The listing builds one solid part. Answer for the finished solid, in the listing's coordinates (mm). Face numbers are marked on the shaded views. A direction names the side the tool comes from. Give positions to 0.01 mm unless a question says otherwise; leave off trailing zeros. Order: outer loops, then holes, each group sorted by start corner. A loop starts at its lowest first (then second) coordinate and runs counter-clockwise, first axis right, second up. Notation, with made-up numbers: (49.25, -40) - (77.25, -40) arc R22 cw to (77.25, -7) - close; hole circle Ø7 at (61, 35.5). An arc over 180 degrees is marked (long way). Write each question's results on one line, items separated by ' | '. Start each with the question number.
1. Flat-ended cylindrical pins translate along their axes: pin 1 (5 mm diameter, centred on x = -16, y = -20, fed in from +Z); pin 2 (4 mm diameter, centred on x = -14.5, z = 6, fed in from +Y); pin 3 (9 mm diameter, centred on x = -18, y = 18.5, fed in from +Z). Find the tip coordinate at first contact, or state that the pin passes through.
2. Section D-D (z = 8) is taken. Give the vertices of the cut face in (x, y), and give its area (3 significant figures).
3. Section B-B (x = 0) is taken. Give the vertices of the cut face in (y, z) (3 decimals).
4. Which of the six approach directions +Z, -Z, +X, -X, +Y, -Y give full straight-line access (tool end or side, diameter ignored) to the marked faces 1, 2, 3 and 4?
5. Find the intervals of material crossed by L1, parallel to Z at x = 9.5, y = 21; L2, parallel to Z at x = -10, y = 1 (3 decimals); L3, parallel to Z at x = 23, y = -5, in increasing order.
6. Determine the mould class of the marked faces 5, 6, 7 and 8 for opening direction Z: released by +Z, released by -Z, zero draft, split by the parting line, or undercut.
7. Section A-A (z = 0) is taken. Give the vertices of the cut face in (x, y) (3 decimals).
8. Section C-C (y = 14) is taken. Give the vertices of the cut face in (x, z), and give its area (3 significant figures).
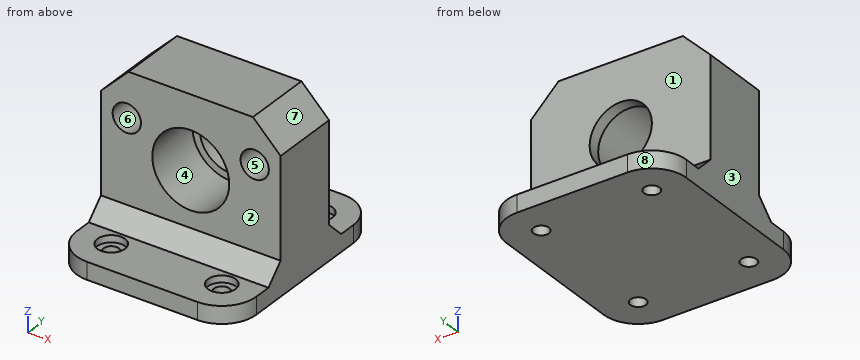
from build123d import *

# Parameters (mm, degrees)
F0_W      = 52
F0_H      = 42
F1_DEPTH  = 10
F2_W      = 52
F2_H      = 5
F3_DEPTH  = 30
F4_R      = 9
F5_DEPTH  = 40.001
F6_R      = 11.125
F6_R_2    = 4.1
F7_DEPTH  = 16.5
F8_R      = 2.25
F9_DEPTH  = 5.001
F10_R     = 4
F11_DEPTH = 2
F12_SIZE  = 8
F13_SIZE  = 5
F14_R     = 10


with BuildPart() as f1:
    # F0 (on Front) → F1 (new body, symmetric)
    with BuildSketch(Plane.XZ):
        Rectangle(F0_W, F0_H)
    extrude(amount=F1_DEPTH, both=True)

    # F2 (on Front) → F3 (join, symmetric)
    with BuildSketch(Plane.XZ):
        with Locations((0, -23.5)):
            Rectangle(F2_W, F2_H)
    extrude(amount=F3_DEPTH, both=True)

    # F4 (on face) → F5 (cut, through all)
    with BuildSketch(Plane.XZ.offset(10)):
        Circle(F4_R)
    extrude(amount=-F5_DEPTH, mode=Mode.SUBTRACT)

    # F6 (on face) → F7 (cut)
    with BuildSketch(Plane.XZ.offset(10)):
        Circle(F6_R)
        with Locations((-18.5, 8)):
            Circle(F6_R_2)
        with Locations((18.5, 8)):
            Circle(F6_R_2)
    extrude(amount=-F7_DEPTH, mode=Mode.SUBTRACT)

    # F8 (on face) → F9 (cut, through all)
    with BuildSketch(Plane.XY.offset(-21)):
        with Locations((-16, 20)):
            Circle(F8_R)
        with Locations((16, 20)):
            Circle(F8_R)
        with Locations((16, -20)):
            Circle(F8_R)
        with Locations((-16, -20)):
            Circle(F8_R)
    extrude(amount=-F9_DEPTH, mode=Mode.SUBTRACT)

    # F10 (on face) → F11 (cut)
    with BuildSketch(Plane.XY.offset(-21)):
        with Locations((-16, 20)):
            Circle(F10_R)
        with Locations((16, 20)):
            Circle(F10_R)
        with Locations((-16, -20)):
            Circle(F10_R)
        with Locations((16, -20)):
            Circle(F10_R)
    extrude(amount=-F11_DEPTH, mode=Mode.SUBTRACT)

    # F12
    f12_edges = [f1.edges().sort_by_distance(p)[0] for p in [
        (-26, 0, 21),
        (26, 0, 21),
    ]]
    chamfer(f12_edges, length=F12_SIZE)

    # F13
    f13_edges = [f1.edges().sort_by_distance(p)[0] for p in [
        (0, -10, -21),
        (0, 10, -21),
    ]]
    chamfer(f13_edges, length=F13_SIZE)

    # F14
    f14_edges = [f1.edges().sort_by_distance(p)[0] for p in [
        (26, 30, -23.5),
        (-26, 30, -23.5),
        (26, -30, -23.5),
        (-26, -30, -23.5),
    ]]
    fillet(f14_edges, radius=F14_R)


solid = f1.part
Reported:
1) pin 1: z = -23 | pin 2: y = 10 | pin 3: z = -20
2) outline: (-26, -10) - (-22.6, -10) - (-22.6, 6.5) - (-14.4, 6.5) - (-14.4, -10) - (-7.73, -10) - (-7.73, 6.5) - (-4.12, 6.5) - (-4.12, 10) - (-26, 10) - close; (4.12, 6.5) - (7.73, 6.5) - (7.73, -10) - (14.4, -10) - (14.4, 6.5) - (22.6, 6.5) - (22.6, -10) - (26, -10) - (26, 10) - (4.12, 10) - close | area: 485 mm²
3) outline: (-30, -26) - (30, -26) - (30, -21) - (15, -21) - (10, -16) - (10, -9) - (6.5, -9) - (6.5, -11.125) - (-10, -11.125) - (-10, -16) - (-15, -21) - (-30, -21) - close; (-10, 11.125) - (6.5, 11.125) - (6.5, 9) - (10, 9) - (10, 21) - (-10, 21) - close
4) face 1: +Z, +X, -X, +Y | face 2: +Z, +X, -X, -Y | face 3: +Z, -Z, -X, +Y, -Y | face 4: -Y
5) L1: -26 to -21 | L2: -26 to -4.875, 4.875 to 21 | L3: -26 to 16
6) face 5: undercut | face 6: undercut | face 7: released by +Z | face 8: zero draft
7) outline: (-26, -10) - (-11.125, -10) - (-11.125, 6.5) - (-9, 6.5) - (-9, 10) - (-26, 10) - close; (9, 6.5) - (11.125, 6.5) - (11.125, -10) - (26, -10) - (26, 10) - (9, 10) - close
8) outline: (-26, -26) - (26, -26) - (26, -20) - (-26, -20) - close | area: 312 mm²
